```python
from build123d import *

# Parameters (mm, degrees)
SKETCH1_W          = 50.8
SKETCH1_H          = 28.575
EXTRUDE1_DEPTH     = 46.7868
SKETCH5_R          = 13.5001
EXTRUDE2_DEPTH     = 5.969
SKETCH6_W          = 6.35
SKETCH6_H          = 10.541
CUT_EXTRUDE4_DEPTH = 30.48
HOLE1_D            = 7.1374
HOLE1_DEPTH        = 46.7868
HOLE2_D            = 7.1374
HOLE2_DEPTH        = 28.575


with BuildPart() as part:
    # Sketch1 → Extrude1 (new body)
    with BuildSketch(Plane(origin=(0, 0, 0), x_dir=(0, 0, -1), z_dir=(1, 0, 0))):
        with Locations((2.3876, 0)):
            Rectangle(SKETCH1_W, SKETCH1_H)
    extrude(amount=EXTRUDE1_DEPTH)

    # S2D0002 → Cut-Revolve1 (revolve, cut)
    with BuildSketch(Plane(origin=(0, 4.7625, 0), x_dir=(-1, 0, 0), z_dir=(0, 1, 0)), mode=Mode.PRIVATE) as cut_revolve1_sk:
        Polygon((-15.7099, -27.5336), (-19.0499873, -27.5336), (-19.0499873, -27.7876), (-9.525, -27.7876), (-9.525, -13.5636), (-14.5034, -13.5636), (-14.5034, -24.316993135), (-15.167306865, -24.9809), align=None)
    revolve(cut_revolve1_sk.sketch.rotate(Axis((9.525, 4.7625, -19.13842003), (0, 0, 1)), 180), axis=Axis((9.525, 4.7625, -19.13842003), (0, 0, 1)), mode=Mode.SUBTRACT)  # turned: the seam where the file's is

    # Sketch3 → Cut-Revolve2 (revolve, cut)
    with BuildSketch(Plane(origin=(41.148, 4.7625, -25.146), x_dir=(1, 0, 0), z_dir=(0, 1, 0))):
        Polygon((2.5019, 2.3876), (5.8419873, 2.3876), (5.8419873, 2.6416), (-3.683, 2.6416), (-3.683, -11.5824), (1.2954, -11.5824), (1.2954, -0.829006865), (1.959306865, -0.1651), align=None)
    revolve(axis=Axis((37.465, 4.7625, -3.189624441), (0, 0, -1)), mode=Mode.SUBTRACT)

    # Sketch5 → Extrude2 (add)
    with BuildSketch(Plane.ZY):
        Circle(SKETCH5_R)
    extrude(amount=EXTRUDE2_DEPTH)

    # Sketch6 → Revolve1 (revolve)
    with BuildSketch(Plane(origin=(0, 0, 0), x_dir=(0, 0, 1), z_dir=(0, -1, 0)), mode=Mode.PRIVATE) as revolve1_sk:
        with Locations((-3.175, 11.2395)):
            Rectangle(SKETCH6_W, SKETCH6_H)
    revolve(revolve1_sk.sketch.rotate(Axis((5.754582971, 0, 0), (-1, 0, 0)), 180), axis=Axis((5.754582971, 0, 0), (-1, 0, 0)))  # turned: the seam where the file's is

    # S2D0001 → Cut-Revolve4 (revolve, cut)
    with BuildSketch(Plane(origin=(-18.511260017, 3.2639, 0), x_dir=(0, 1, 0), z_dir=(0, 0, 1)), mode=Mode.PRIVATE) as cut_revolve4_sk:
        Polygon((-0.7112, -3.563050231), (-0.7112, -18.003260017), (-3.2639, -19.53707692), (-3.2639, -2.001260017), (0.1905, -2.001260017), align=None)
    revolve(cut_revolve4_sk.sketch.rotate(Axis((0, 0, 0), (-1, 0, 0)), 90), axis=Axis((0, 0, 0), (-1, 0, 0)), mode=Mode.SUBTRACT)  # turned: the seam where the file's is

    # Sketch8 → Cut-Revolve5 (revolve, cut)
    with BuildSketch(Plane(origin=(0, 0, 0), x_dir=(0, 0, -1), z_dir=(0, 1, 0)), mode=Mode.PRIVATE) as cut_revolve5_sk:
        with BuildLine():
            Line((-6.35, 10.1854), (-6.096, 10.9474))
            Line((-6.096, 10.9474), (-6.096, 15.494))
            ThreePointArc((-6.096, 15.494), (-5.995678675, 16.037796865), (-5.707922533, 16.51))
            Line((-5.707922533, 16.51), (-6.35, 16.51))
            Line((-6.35, 16.51), (-6.35, 10.1854))
        make_face()
    revolve(cut_revolve5_sk.sketch.rotate(Axis((-12.65936, 0, 0), (-1, 0, 0)), 180), axis=Axis((-12.65936, 0, 0), (-1, 0, 0)), mode=Mode.SUBTRACT)  # turned: the seam where the file's is

    # Sketch12 → Cut-Extrude4 (cut, symmetric)
    with BuildSketch(Plane(origin=(0, 0, 0), x_dir=(0, -1, 0), z_dir=(0, 0, -1))):
        Polygon((5.461, 16.51), (5.461, 11.7348), (6.096, 11.0998), (6.096, 16.51), align=None)
        Polygon((-5.461, 16.51), (-5.461, 11.7348), (-6.096, 11.0998), (-6.096, 16.51), align=None)
    extrude(amount=CUT_EXTRUDE4_DEPTH, both=True, mode=Mode.SUBTRACT)

    # Hole1
    with Locations(Plane.ZY):
        with Locations((-16.6878, -7.9248), (16.6624, 7.9502)):
            Hole(HOLE1_D / 2, depth=HOLE1_DEPTH)

    # Hole2
    with Locations(Plane(origin=(0, 14.2875, 0), x_dir=(-1, 0, 0), z_dir=(0, 1, 0))):
        with Locations((-23.3172, -16.6878), (-23.3172, 16.6624)):
            Hole(HOLE2_D / 2, depth=HOLE2_DEPTH)


solid = part.part
```
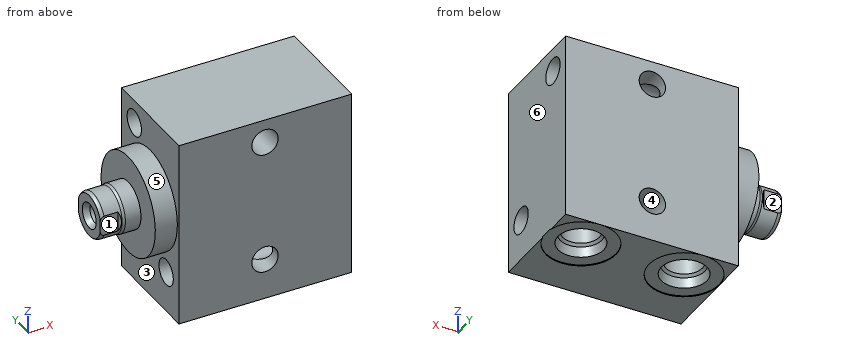
The listing builds one solid part. Answer for the finished solid, in the listing's coordinates (mm). Face numbers are marked on the shaded views. A direction names the side the tool comes from. Give positions to 0.01 mm unless a question says otherwise; leave off trailing zeros. Order: outer loops, then holes, each group sorted by start corner. A loop starts at its lowest first (then second) coordinate and runs counter-clockwise, first axis right, second up. Notation, with made-up numbers: (39.5, 47.5) -> (55.5, 47.5) arc R6 cw to (55.5, 55.5) -> close; hole circle Ø10 at (-36.5, 7). An arc over 180 degrees is marked (long way). Answer as CSV lines item,"result". Start each with the question number.
Q1. Which of the six approach directions +Z, -Z, +X, -X, +Y, -Y give full straight-line access (tool end or side, diameter ignored) to the marked faces 1, 2 and 3?
Q2. Determine the mould class of the marked faces 4, 5 and 6 for opening direction X: pulls with the +X half, pulls with the -X half, needs draft (parallel to the pull), parting line crosses it, or undercut.
Q3. Find the intervals of material crossed by L1, parallel to Z at x = 23, y = -8.5; L2, parallel to X at y = -0.25, z = -17; L3, parallel to X at y = 9.5, z = -13, in increasing order.
Q4. Given pin 1 (5.5 mm diameter, centred on x = 10, y = 8.5, fed in from -Z); pin 2 (6 mm diameter, centred on y = 10.5, z = -6.5, fed in from -X); pin 3 (4 mm diameter, centred on x = -15.5, z = 1.5, fed in from +Y), each flat-ended and moving along its own axis, determine where each tip first touches the part or whether it passes through.
Q5. A cutting plane is placed at B-B (z = -9). Determine the outline of the cut face in (x, y), then the cut area to 3 significant figures.
Q6. A cutting plane is placed at A-A (x = -2). Determine the outline of the cut face in (y, z).
Q7. A cutting plane is placed at C-C (x = 10). Count the separate pieces of the cut face and the enclosed holes in it, then the cut area to 3 significant figures.
Results found:
1,face 1,"+Z, -Z, -X, -Y"
1,face 2,"+Z, -Z, -X, +Y"
1,face 3,"-X"
2,face 4,"undercut"
2,face 5,"needs draft"
2,face 6,"pulls with the +X half"
3,L1,"-27.79 to -20.24, -13.13 to 13.11, 20.22 to 23.01"
3,L2,"0 to 19.76, 26.87 to 46.79"
3,L3,"0 to 46.79"
4,pin 1,"z = -27.53"
4,pin 2,"x = -5.97"
4,pin 3,"y = 5.46"
5,outline,"(-5.97, -10.06) -> (0, -10.06) -> (0, -14.29) -> (46.79, -14.29) -> (46.79, 14.29) -> (0, 14.29) -> (0, 10.06) -> (-5.97, 10.06) -> close"
5,area,"1,460 mm2"
6,outline,"circle Ø27 at (0, 0); hole circle Ø5.11 at (0, 0)"
7,separate pieces,"1"
7,enclosed holes,"2"
7,area,"1,220 mm2"
